Can you work these out from the drawing? Everything is in mm from the part's minimum corner. A direction names the side the tool comes from. Round coordinates to 2 decimals unless told otherwise and drop trailing zeros. Write each loop counter-clockwise with the first axis right and the second up, starting at its lowest first coordinate (ties: lowest second). Pieces come first, ordered by that corner, then holes. Notation, with made-up numbers: M -26,26 L 23,26 A25 ccw 23,49 Z; hole C 21.5,-31 d11. An arc over 180 degrees is marked long. Use a Markdown table: item, result. Add a question column.
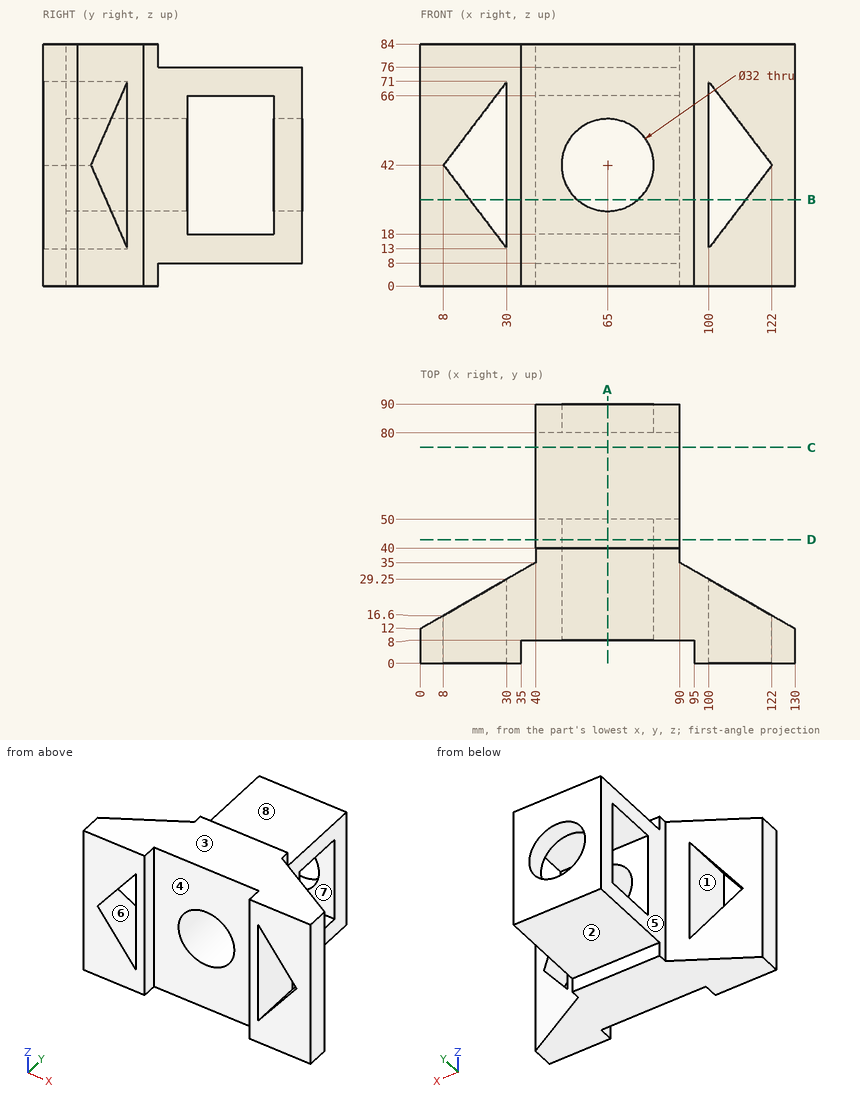
Item 1: Imagine slicing it at A-A on x = 65. List the corners of the cut face in (y, z) for me.
Item 2: I need wall thicknesses on probe 1 along Z at (x, y) = (65, 84.5); probe 2 along Z at (x, y) = (65, 22.5); probe 3 along X at (y, z) = (7, 47.5). Which ranges of each line are inside material? Lowest first, please. Write a range as from..to.
Item 3: On a 3-axis mill with a long thin cutter (end or side, diameter ignored), from which of +Z, -Z, +X, -X, +Y, -Y can I reach the whole of each face in a straight line? I mean the marked faces 4, 5, 6, 7 and 8. Say none if no direction works.
Item 4: Imagine slicing it at B-B on z = 30. Count the separate pieces of the cut face and the enclosed holes in it, plus the area to 3 significant figures.
Item 5: Imagine slicing it at C-C on y = 75. List the corners of the cut face in (x, z) for me.
Item 6: Imagine slicing it at D-D on y = 43. List the corners of the cut face in (x, z) for me.
Item 7: If we mould it in two halves opening along Z, with no side actions, what happens to the marked faces 1, 2 and 3? For each: +Z half, -Z half, draft (parallel to the pull), parting line (faces both ways), or undercut.
Item 8: For pin 1 Ø16.5 at (y, z) = (57.5, 38) entering from +X; pin 2 Ø4 at (y, z) = (2.5, 26.5) entering from -X; pin 3 Ø3 at (y, z) = (28.5, 74.5) entering from -X; pin 4 Ø16.5 at (y, z) = (57, 51.5) entering from -X, each with a flat end and sliding along its axis, tell me the tip position at first contact or that it passes through.
The answers:
| question | item | result |
|---|---|---|
| 1 | outline | M 8,0 L 40,0 L 40,8 L 90,8 L 90,26 L 80,26 L 80,18 L 50,18 L 50,26 L 8,26 Z; M 8,58 L 50,58 L 50,66 L 80,66 L 80,58 L 90,58 L 90,76 L 40,76 L 40,84 L 8,84 Z |
| 2 | probe 1 | 8..26, 58..76 |
| 2 | probe 2 | 0..26, 58..84 |
| 2 | probe 3 | 0..12.17, 30..35, 95..100, 117.83..130 |
| 3 | face 4 | +Z, -Z, -Y |
| 3 | face 5 | +Z, -Z, -X, +Y |
| 3 | face 6 | +Y, -Y |
| 3 | face 7 | +X, -X |
| 3 | face 8 | +Z, +X, -X, +Y |
| 4 | separate pieces | 6 |
| 4 | enclosed holes | 0 |
| 4 | area | 2,640 mm² |
| 5 | outline | M 40,8 L 90,8 L 90,18 L 40,18 Z; M 40,66 L 90,66 L 90,76 L 40,76 Z |
| 6 | outline | M 40,8 L 90,8 L 90,76 L 40,76 Z; hole C 65,42 d32 |
| 7 | face 1 | undercut |
| 7 | face 2 | -Z half |
| 7 | face 3 | +Z half |
| 8 | pin 1 | x = 90 |
| 8 | pin 2 | x = 0 |
| 8 | pin 3 | x = 26.09 |
| 8 | pin 4 | x = 40 |
